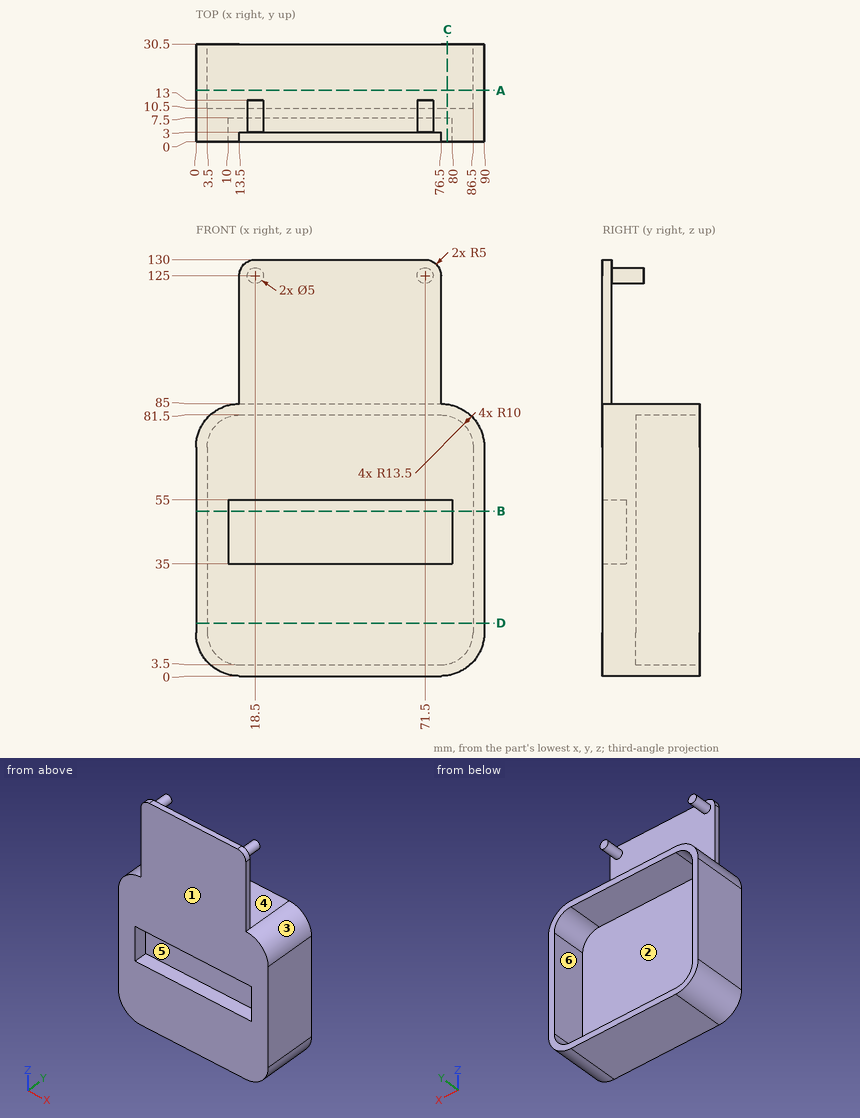
For this review, use the dimensioned drawing (mm, ordinates from the lowest corner) and the shaded views. A direction names the side the tool comes from. Coordinates: 2 decimals unless noted, no trailing zeros. Loops run counter-clockwise (first coordinate to the right, second up) from the corner with the lowest first, then second, coordinate; pieces in that order, holes last.
1. Add section C-C, the plane x = 78.5. Give the boundary of the cut face in (y, z).
2. Mouldability with a two-part tool opening along X and no side actions: class the marked faces 3, 4, 5 and 6 as +X half, -X half, draft (parallel to the pull), parting line (faces both ways), or undercut.
3. Insertion check: P1, Ø6, axis at x = 34, y = 17, coming from the +Z side; P2, Ø1.5, axis at y = 1.5, z = 108, coming from the +X side; P3, Ø6, axis at x = 28, z = 46.5, coming from the -Y side. Each pin has a flat end and moves straight along its axis. Give the tip position at first contact, or say it passes through.
4. For the marked faces 1 and 2, list the 3-axis set-ups (+Z, -Z, +X, -X, +Y, -Y) from which the entire face can be reached by the end or side of a thin tool; tool diameter is ignored.
5. Add section D-D, the plane z = 16.5. Give the boundary of the cut face in (x, y).
6. For line 1 (Z direction, x = 45.5, y = 27.5); line 2 (Y direction, x = 83, z = 43.5); line 3 (Y direction, x = 21.5, z = 52.5), list the stretches that pass through material, from the lowest coordinate up.
7. Add section B-B, the plane z = 51.5. Give the boundary of the cut face in (x, y).
8. Add section A-A, the plane y = 16. Give the boundary of the cut face in (x, z), then the cut area to 3 significant figures.
Result:
1. outline: (0, 0.15) - (30.5, 0.15) - (30.5, 3.7) - (10.5, 3.7) - (10.5, 81.3) - (30.5, 81.3) - (30.5, 84.85) - (0, 84.85) - (0, 55) - (7.5, 55) - (7.5, 35) - (0, 35) - close
2. face 3: +X half
2. face 4: draft
2. face 5: undercut
2. face 6: undercut
3. P1: stops at z = 85
3. P2: stops at x = 76.5
3. P3: stops at y = 7.5
4. face 1: +Z, -Z, +X, -X, -Y
4. face 2: +Y
5. outline: (0, 0) - (90, 0) - (90, 30.5) - (86.5, 30.5) - (86.5, 10.5) - (3.5, 10.5) - (3.5, 30.5) - (0, 30.5) - close
6. line 1: z = 0 to 3.5, 81.5 to 85
6. line 2: y = 0 to 10.5
6. line 3: y = 7.5 to 10.5
7. outline: (0, 0) - (10, 0) - (10, 7.5) - (80, 7.5) - (80, 0) - (90, 0) - (90, 30.5) - (86.5, 30.5) - (86.5, 10.5) - (3.5, 10.5) - (3.5, 30.5) - (0, 30.5) - close
8. outline: (0, 13.5) arc R13.5 ccw to (13.5, 0) - (76.5, 0) arc R13.5 ccw to (90, 13.5) - (90, 71.5) arc R13.5 ccw to (76.5, 85) - (13.5, 85) arc R13.5 ccw to (0, 71.5) - close; hole (3.5, 13.5) arc R10 ccw to (13.5, 3.5) - (76.5, 3.5) arc R10 ccw to (86.5, 13.5) - (86.5, 71.5) arc R10 ccw to (76.5, 81.5) - (13.5, 81.5) arc R10 ccw to (3.5, 71.5) - close
8. area: 1,110 mm2
